Part model, mm, in its own coordinate system. A direction names the side the tool comes from. Round coordinates to 2 decimals unless told otherwise and drop trailing zeros. Write each loop counter-clockwise with the first axis right and the second up, starting at its lowest first coordinate (ties: lowest second). Pieces come first, ordered by that corner, then holes.
1) Flat gauge pins, fed straight in: pin 1 (0.9 mm diameter, centred on x = 0, y = 1, fed in from +Z); pin 2 (3 mm diameter, centred on x = 12.5, z = -20.5, fed in from -Y). Where does each tip first touch, or does it go through?
2) Saw through at A-A on z = -13.5. Write the cut outline in (x, y), and give its area (3 significant figures).
3) Drill centre lines: L1, parallel to X at y = 1, z = -13.5; L2, parallel to X at y = 0.5, z = -17.5; L3, parallel to X at y = 1.5, z = -26. Where is each one in solid material? Low to high.
4) Pull direction Z, two halves, no side cores. Call faces 6 (the flat face through (14, 11.5, -43)), 7 (the flat face through (0, 1, 6.104)), 8 (the flat face through (0, 1, -25.896)): +Z half, -Z half, draft (parallel to the pull), parting line (faces both ways), or undercut.
5) Saw through at C-C on x = -10.5. Write the cut outline in (y, z), and give its area (3 significant figures).
6) Saw through at D-D on z = -1.5. Write the cut outline in (x, y).
7) Which spindle directions (+Z, -Z, +X, -X, +Y, -Y) get a long thin tool onto all of the face, cutting with end or side? Do faces 1 (the flat face through (0, 1, -17.896)), 2 (the cylindrical face through (9.03, 1.479, -3.563)), 3 (the cylindrical face through (14.27, 4.14, 9.49)), 4 (the cylindrical face through (14.229, 8.458, -40.586)), 5 (the flat face through (12.75, 5, -41)). Say none if no direction does.
8) Saw through at B-B on y = 8.5. Count the separate pieces of the cut face and the enclosed holes in it, and give its area (3 significant figures).
```python
from build123d import *

# Parameters (mm, degrees)
SKETCH1_W               = 54
SKETCH1_H               = 3
BOSS_EXTRUDE1_DEPTH     = 12.75
SKETCH2_W               = 3
SKETCH2_H               = 68.59
BOSS_EXTRUDE2_DEPTH     = 3
SKETCH4_R               = 2.1
CUT_EXTRUDE2_DEPTH      = 3
SKETCH5_W               = 3
SKETCH5_H               = 10
BOSS_EXTRUDE3_DEPTH     = 8.5
SKETCH6_W               = 31.5
SKETCH6_H               = 8
CUT_EXTRUDE3_DEPTH      = 2
FILLET1_R               = 4
CUT_EXTRUDE4_DEPTH      = 52.130188209
CUT_EXTRUDE4_DEPTH_BACK = 52.130188209
CUT_EXTRUDE5_DEPTH      = 59.46780008
CUT_EXTRUDE5_DEPTH_BACK = 59.46780008
SKETCH8_R               = 2.5


with BuildPart() as part:
    # Sketch1 → Boss-Extrude1 (new, symmetric)
    with BuildSketch(Plane(origin=(0, 0, 0), x_dir=(0, 0, -1), z_dir=(1, 0, 0))):
        with Locations((20.895549337, 1.5)):
            Rectangle(SKETCH1_W, SKETCH1_H)
    extrude(amount=BOSS_EXTRUDE1_DEPTH, both=True)

    # Sketch2 → Boss-Extrude2 (add)
    with BuildSketch(Plane(origin=(0, 0, 0), x_dir=(1, 0, 0), z_dir=(0, 1, 0))):
        with Locations((14.25, 13.600549337)):
            Rectangle(SKETCH2_W, SKETCH2_H)
        with Locations((-14.25, 13.600549337)):
            Rectangle(SKETCH2_W, SKETCH2_H)
    extrude(amount=BOSS_EXTRUDE2_DEPTH)

    # Sketch4 → Cut-Extrude2 (cut)
    with BuildSketch(Plane(origin=(0, 3, 0), x_dir=(1, 0, 0), z_dir=(0, 1, 0))):
        with Locations(Location((0, 13.5, 0), (0, 0, 270))):
            Circle(SKETCH4_R)
        with BuildLine():
            ThreePointArc((0.510375011, 28.172498171), (1.842935069, 29.202762349), (1.989848247, 30.880730496))
            ThreePointArc((1.989848247, 30.880730496), (0.567559264, 32.231384351), (-1.34985398, 31.818227914))
            ThreePointArc((-1.34985398, 31.818227914), (-1.870566111, 29.255080591), (0.510375011, 28.172498171))
        make_face()
    extrude(amount=-CUT_EXTRUDE2_DEPTH, mode=Mode.SUBTRACT)

    # Sketch5 → Boss-Extrude3 (add)
    with BuildSketch(Plane(origin=(0, 3, 0), x_dir=(1, 0, 0), z_dir=(0, 1, 0))):
        with Locations((-14.25, -15.694450663)):
            Rectangle(SKETCH5_W, SKETCH5_H)
        with Locations((14.25, -15.694450663)):
            Rectangle(SKETCH5_W, SKETCH5_H)
        with Locations((14.25, 42.895549337)):
            Rectangle(SKETCH5_W, SKETCH5_H)
        with Locations((-14.25, 42.895549337)):
            Rectangle(SKETCH5_W, SKETCH5_H)
    extrude(amount=BOSS_EXTRUDE3_DEPTH)

    # Sketch6 → Cut-Extrude3 (cut)
    with BuildSketch(Plane.XZ):
        with Locations((0, -21.895549337)):
            Rectangle(SKETCH6_W, SKETCH6_H)
    extrude(amount=-CUT_EXTRUDE3_DEPTH, mode=Mode.SUBTRACT)

    # Fillet1
    fillet1_edges = [part.edges().sort_by_distance(p)[0] for p in [
        (-14.25, 3, -37.895549337),
        (-14.25, 11.5, -47.895549337),
        (-14.25, 11.5, -37.895549337),
        (14.25, 3, -37.895549337),
        (14.25, 11.5, -37.895549337),
        (14.25, 11.5, -47.895549337),
        (14.25, 3, 10.694450663),
        (14.25, 11.5, 20.694450663),
        (14.25, 11.5, 10.694450663),
        (-14.25, 3, 10.694450663),
        (-14.25, 11.5, 10.694450663),
        (-14.25, 11.5, 20.694450663),
    ]]
    fillet(fillet1_edges, radius=FILLET1_R)

    # Sketch7 → Cut-Extrude4 (cut, two sides: drawn at the far end of the back side and taken through both)
    with BuildSketch(Plane(origin=(0, 3, 0), x_dir=(1, 0, 0), z_dir=(0, 1, 0)).offset(-CUT_EXTRUDE4_DEPTH_BACK)):
        with BuildLine():
            Line((0.964735196, 7.90721125), (6.54617705, -1.598099098))
            ThreePointArc((6.54617705, -1.598099098), (6.551706918, -2.60126473), (5.683849912, -3.104450663))
            Line((5.683849912, -3.104450663), (-5.683849912, -3.104450663))
            ThreePointArc((-5.683849912, -3.104450663), (-6.551706918, -2.60126473), (-6.54617705, -1.598099098))
            Line((-6.54617705, -1.598099098), (-0.964735196, 7.90721125))
            ThreePointArc((-0.964735196, 7.90721125), (-0.591919483, 8.272856568), (-0.085619852, 8.400718753))
            ThreePointArc((-0.085619852, 8.400718753), (0, 8.4), (0.085619852, 8.400718753))
            ThreePointArc((0.085619852, 8.400718753), (0.591919483, 8.272856568), (0.964735196, 7.90721125))
        make_face()
        with BuildLine():
            Line((-4.603921215, 33.528255639), (-7.916886234, 38.518435448))
            ThreePointArc((-7.916886234, 38.518435448), (-9.038865223, 38.922703555), (-9.75, 37.965333782))
            Line((-9.75, 37.965333782), (-9.75, 4.523307202))
            ThreePointArc((-9.75, 4.523307202), (-9.012366978, 3.558339032), (-7.887672863, 4.016955636))
            Line((-7.887672863, 4.016955636), (-4.414043746, 9.932617513))
            ThreePointArc((-4.414043746, 9.932617513), (-4.276374342, 10.436338854), (-4.41139205, 10.940777426))
            ThreePointArc((-4.41139205, 10.940777426), (-4.921337666, 14.838071589), (-2.508196721, 17.940602347))
            ThreePointArc((-2.508196721, 17.940602347), (-2.136344027, 18.30722699), (-2, 18.81130869))
            Line((-2, 18.81130869), (-2, 24.898225894))
            ThreePointArc((-2, 24.898225894), (-2.136344027, 25.402307594), (-2.508196721, 25.768932236))
            ThreePointArc((-2.508196721, 25.768932236), (-4.882585845, 28.736321948), (-4.545717772, 32.521773745))
            ThreePointArc((-4.545717772, 32.521773745), (-4.438702873, 33.032886126), (-4.603921215, 33.528255639))
        make_face()
        with BuildLine():
            Line((1.27146615, 35.740662301), (6.318268064, 43.342447671))
            ThreePointArc((6.318268064, 43.342447671), (6.366375514, 44.368253438), (5.485154298, 44.895549337))
            Line((5.485154298, 44.895549337), (-5.485154298, 44.895549337))
            ThreePointArc((-5.485154298, 44.895549337), (-6.366375514, 44.368253438), (-6.318268064, 43.342447671))
            Line((-6.318268064, 43.342447671), (-1.27146615, 35.740662301))
            ThreePointArc((-1.27146615, 35.740662301), (-0.879067636, 35.396117006), (-0.366491338, 35.296349314))
            ThreePointArc((-0.366491338, 35.296349314), (0, 35.309534584), (0.366491338, 35.296349314))
            ThreePointArc((0.366491338, 35.296349314), (0.879067636, 35.396117006), (1.27146615, 35.740662301))
        make_face()
        with BuildLine():
            Line((4.603921215, 33.528255639), (7.916886234, 38.518435448))
            ThreePointArc((7.916886234, 38.518435448), (9.038865223, 38.922703555), (9.75, 37.965333782))
            Line((9.75, 37.965333782), (9.75, 4.523307202))
            ThreePointArc((9.75, 4.523307202), (9.012366978, 3.558339032), (7.887672863, 4.016955636))
            Line((7.887672863, 4.016955636), (4.414043746, 9.932617513))
            ThreePointArc((4.414043746, 9.932617513), (4.276374342, 10.436338854), (4.41139205, 10.940777426))
            ThreePointArc((4.41139205, 10.940777426), (4.921337666, 14.838071589), (2.508196721, 17.940602347))
            ThreePointArc((2.508196721, 17.940602347), (2.136344027, 18.30722699), (2, 18.81130869))
            Line((2, 18.81130869), (2, 24.898225894))
            ThreePointArc((2, 24.898225894), (2.136344027, 25.402307594), (2.508196721, 25.768932236))
            ThreePointArc((2.508196721, 25.768932236), (4.882585845, 28.736321948), (4.545717772, 32.521773745))
            ThreePointArc((4.545717772, 32.521773745), (4.438702873, 33.032886126), (4.603921215, 33.528255639))
        make_face()
    extrude(amount=CUT_EXTRUDE4_DEPTH + CUT_EXTRUDE4_DEPTH_BACK, mode=Mode.SUBTRACT)

    # Sketch8 → Cut-Extrude5 (cut, two sides: drawn at the far end of the back side and taken through both)
    with BuildSketch(Plane(origin=(15.75, 0, 0), x_dir=(0, 0, -1), z_dir=(1, 0, 0)).offset(-CUT_EXTRUDE5_DEPTH_BACK)):
        with Locations((-15.694450663, 7.5)):
            Circle(SKETCH8_R)
        with Locations(Location((42.895549337, 7.5, 0), (0, 0, 180))):
            Circle(SKETCH8_R)
    extrude(amount=CUT_EXTRUDE5_DEPTH + CUT_EXTRUDE5_DEPTH_BACK, mode=Mode.SUBTRACT)


solid = part.part
```
Completed:
1. pin 1: stops at z = 6.1
1. pin 2: stops at y = 2
2. outline: (-15.75, 0) - (-9.75, 0) - (-9.75, 3) - (-15.75, 3) - close; (-5.1, 0) - (-2.1, 0) - (-2.1, 3) - (-5.1, 3) - close; (2.1, 0) - (5.1, 0) - (5.1, 3) - (2.1, 3) - close; (9.75, 0) - (15.75, 0) - (15.75, 3) - (9.75, 3) - close
2. area: 54.0 mm2
3. L1: x = -15.75 to -9.75, -5.1 to -2.1, 2.1 to 5.1, 9.75 to 15.75
3. L2: x = -15.75 to -9.75, -3.16 to 3.16, 9.75 to 15.75
3. L3: x = -15.75 to -9.75, -2.88 to 2.88, 9.75 to 15.75
4. face 6: draft
4. face 7: +Z half
4. face 8: undercut
5. outline: (0, -47.9) - (3, -47.9) - (3, 6.1) - (0, 6.1) - (0, -17.9) - (2, -17.9) - (2, -25.9) - (0, -25.9) - close
5. area: 146 mm2
6. outline: (-15.75, 0) - (-4.73, 0) - (-4.73, 3) - (-15.75, 3) - close; (4.73, 0) - (15.75, 0) - (15.75, 3) - (4.73, 3) - close
7. face 1: +X, -X, -Y
7. face 2: +Y, -Y
7. face 3: +X, -X, +Y
7. face 4: +X, -X
7. face 5: +Z, -Z, +Y
8. separate pieces: 8
8. enclosed holes: 0
8. area: 62.0 mm2
